```python
from build123d import *

# Parameters (mm, degrees)
SKETCH1_W           = 25
SKETCH1_H           = 25
SKETCH1_W_2         = 22
SKETCH1_H_2         = 22
BOSS_EXTRUDE1_DEPTH = 310
SKETCH2_W           = 25
SKETCH2_H           = 25
SKETCH2_W_2         = 22
SKETCH2_H_2         = 22
BOSS_EXTRUDE2_DEPTH = 30
SKETCH8_R           = 5
CUT_EXTRUDE1_DEPTH  = 25
SKETCH9_R           = 18
SKETCH9_R_2         = 5
BOSS_EXTRUDE3_DEPTH = 10
SKETCH10_R          = 18
SKETCH10_R_2        = 5
BOSS_EXTRUDE4_DEPTH = 10
SKETCH11_W          = 12
SKETCH11_H          = 10
CUT_EXTRUDE2_DEPTH  = 5


with BuildPart() as part:
    # Sketch1 → Boss-Extrude1 (new body)
    with BuildSketch(Plane(origin=(0, 0, 0), x_dir=(1, 0, 0), z_dir=(0, 1, 0))):
        with Locations((30.5, -0.057992327)):
            Rectangle(SKETCH1_W, SKETCH1_H)
        with Locations((30.5, -0.057992327)):
            Rectangle(SKETCH1_W_2, SKETCH1_H_2, mode=Mode.SUBTRACT)
    boss_extrude1 = extrude(amount=BOSS_EXTRUDE1_DEPTH)

    # Sketch2 → Boss-Extrude2 (add)
    # profile 1 of 2: a face of its own
    with BuildSketch(Plane.ZY.offset(-18)):
        with Locations((0.057992327, 197.5)):
            Rectangle(SKETCH2_W, SKETCH2_H)
        with Locations((0.057992327, 197.5)):
            Rectangle(SKETCH2_W_2, SKETCH2_H_2, mode=Mode.SUBTRACT)
    # profile 2 of 2: a face of its own
    with BuildSketch(Plane.ZY.offset(-18)):
        with Locations((0.057992327, 112.5)):
            Rectangle(SKETCH2_W, SKETCH2_H)
        with Locations((0.057992327, 112.5)):
            Rectangle(SKETCH2_W_2, SKETCH2_H_2, mode=Mode.SUBTRACT)
    boss_extrude2 = extrude(amount=BOSS_EXTRUDE2_DEPTH)

    # Sketch8 → Cut-Extrude1 (cut)
    with BuildSketch(Plane.ZY.offset(-18)):
        with Locations((0, 280)):
            Circle(SKETCH8_R)
        with Locations((0, 30)):
            Circle(SKETCH8_R)
    cut_extrude1 = extrude(amount=-CUT_EXTRUDE1_DEPTH, mode=Mode.SUBTRACT)

    # Sketch9 → Boss-Extrude3 (add)
    # profile 1 of 3: a face of its own
    with BuildSketch(Plane(origin=(43, 0, 0), x_dir=(0, 0, -1), z_dir=(1, 0, 0))):
        with Locations((0, 30)):
            Circle(SKETCH9_R)
        with Locations(Location((0, 30, 0), (0, 0, 180))):
            Circle(SKETCH9_R_2, mode=Mode.SUBTRACT)
    # profile 2 of 3: a face of its own
    with BuildSketch(Plane(origin=(43, 0, 0), x_dir=(0, 0, -1), z_dir=(1, 0, 0))):
        with BuildLine():
            Line((-6, 13.029437252), (-6, 3.029437252))
            Line((-6, 3.029437252), (6, 3.029437252))
            Line((6, 3.029437252), (6, 13.029437252))
            ThreePointArc((6, 13.029437252), (0, 12), (-6, 13.029437252))
        make_face()
    # profile 3 of 3: a face of its own
    with BuildSketch(Plane(origin=(43, 0, 0), x_dir=(0, 0, -1), z_dir=(1, 0, 0))):
        with BuildLine():
            Line((-6, 46.970562748), (-6, 56.970562748))
            Line((-6, 56.970562748), (6, 56.970562748))
            Line((6, 56.970562748), (6, 46.970562748))
            ThreePointArc((6, 46.970562748), (0, 48), (-6, 46.970562748))
        make_face()
    boss_extrude3 = extrude(amount=BOSS_EXTRUDE3_DEPTH)

    # Sketch10 → Boss-Extrude4 (add)
    # profile 1 of 3: a face of its own
    with BuildSketch(Plane(origin=(43, 0, 0), x_dir=(0, 0, -1), z_dir=(1, 0, 0))):
        with Locations((0, 280)):
            Circle(SKETCH10_R)
        with Locations(Location((0, 280, 0), (0, 0, 180))):
            Circle(SKETCH10_R_2, mode=Mode.SUBTRACT)
    # profile 2 of 3: a face of its own
    with BuildSketch(Plane(origin=(43, 0, 0), x_dir=(0, 0, -1), z_dir=(1, 0, 0))):
        with BuildLine():
            Line((-6, 296.970562748), (-6, 306.970562748))
            Line((-6, 306.970562748), (6, 306.970562748))
            Line((6, 306.970562748), (6, 296.970562748))
            ThreePointArc((6, 296.970562748), (0, 298), (-6, 296.970562748))
        make_face()
    # profile 3 of 3: a face of its own
    with BuildSketch(Plane(origin=(43, 0, 0), x_dir=(0, 0, -1), z_dir=(1, 0, 0))):
        with BuildLine():
            Line((-6, 263.029437252), (-6, 253.029437252))
            Line((-6, 253.029437252), (6, 253.029437252))
            Line((6, 253.029437252), (6, 263.029437252))
            ThreePointArc((6, 263.029437252), (0, 262), (-6, 263.029437252))
        make_face()
    boss_extrude4 = extrude(amount=BOSS_EXTRUDE4_DEPTH)

    # Sketch11 → Cut-Extrude2 (cut)
    with BuildSketch(Plane(origin=(53, 0, 0), x_dir=(0, 0, -1), z_dir=(1, 0, 0))):
        with Locations((0, 8.029437252)):
            Rectangle(SKETCH11_W, SKETCH11_H)
        with Locations((0, 51.970562748)):
            Rectangle(SKETCH11_W, SKETCH11_H)
        with Locations((0, 258.029437252)):
            Rectangle(SKETCH11_W, SKETCH11_H)
        with Locations((0, 301.970562748)):
            Rectangle(SKETCH11_W, SKETCH11_H)
    cut_extrude2 = extrude(amount=-CUT_EXTRUDE2_DEPTH, mode=Mode.SUBTRACT)

    # Mirror1: Boss-Extrude1, Boss-Extrude2, Cut-Extrude1, Boss-Extrude3, Boss-Extrude4, Cut-Extrude2 across plane
    add(boss_extrude1.mirror(Plane.ZY.offset(12)))
    add(boss_extrude2.mirror(Plane.ZY.offset(12)))
    add(cut_extrude1.mirror(Plane.ZY.offset(12)), mode=Mode.SUBTRACT)
    add(boss_extrude3.mirror(Plane.ZY.offset(12)))
    add(boss_extrude4.mirror(Plane.ZY.offset(12)))
    add(cut_extrude2.mirror(Plane.ZY.offset(12)), mode=Mode.SUBTRACT)


solid = part.part
```
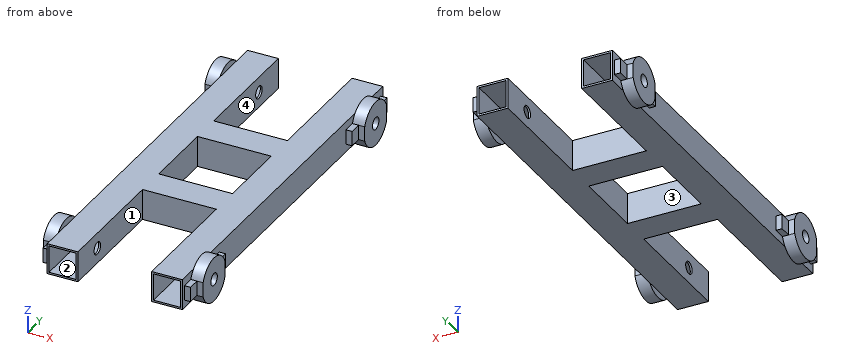
Could you check a few things on this model? Use its own coordinates, in mm. Face numbers are marked on the shaded views. A direction names the side the tool comes from. Coordinates: 2 decimals unless noted, no trailing zeros. Write each loop counter-clockwise with the first axis right and the second up, starting at its lowest first coordinate (ties: lowest second). Pieces come first, ordered by that corner, then holes. Notation, with made-up numbers: (-3.75, -23) -> (47.25, -23) arc R37 ccw to (47.25, 14) -> close; hole circle Ø1 at (58, 20.25). An arc over 180 degrees is marked (long way). Write item = value, one per line. Start each with the question number.
(1) Will these pins go through, and if not, where does the flat tip stop? pin 1 (17.5 mm diameter, centred on y = 196.5, z = 5, fed in from -X); pin 2 (4 mm diameter, centred on x = -33.5, z = 12.5, fed in from -Y); pin 3 (1.5 mm diameter, centred on x = -69.5, z = 0, fed in from +Y).
(2) I want a section at B-B (x = 10.5). Please give me the cut outline in (y, z), plus the area to 3 significant figures.
(3) I need wall thicknesses on line 1 (Y direction, x = -40.5, z = 1); line 2 (X direction, y = 203, z = 5); line 3 (X direction, y = 290, z = 7.5). Which ranges of each line are inside material? Lowest first, please. Write a range as [from, to].
(4) I want a section at A-A (y = 237). Please give me the cut outline in (x, z).
(5) Which directions (+Z, -Z, +X, -X, +Y, -Y) give clear straight access to the entire face, cutting with the end or side of a thin tool? Please do the marked faces 1, 2, 3 and 4.
(6) I want a section at C-C (z = 0). Give the number of separate pieces and of enclosed holes in the cut face, plus the area to 3 significant figures.
Result set:
q1.pin_1 = -67
q1.pin_2 = 100
q1.pin_3 = 306.97
q2.outline = (100, -12.44) -> (125, -12.44) -> (125, 12.56) -> (100, 12.56) -> close; (185, -12.44) -> (210, -12.44) -> (210, 12.56) -> (185, 12.56) -> close; hole (101.5, -10.94) -> (123.5, -10.94) -> (123.5, 11.06) -> (101.5, 11.06) -> close; hole (186.5, -10.94) -> (208.5, -10.94) -> (208.5, 11.06) -> (186.5, 11.06) -> close
q2.area = 282 mm2
q3.line_1 = [100, 101.5], [123.5, 125], [185, 186.5], [208.5, 210]
q3.line_2 = [-67, -65.5], [-43.5, -42], [18, 19.5], [41.5, 43]
q3.line_3 = [-77, -65.5], [-43.5, -42], [18, 19.5], [41.5, 53]
q4.outline = (-67, -12.44) -> (-42, -12.44) -> (-42, 12.56) -> (-67, 12.56) -> close; (18, -12.44) -> (43, -12.44) -> (43, 12.56) -> (18, 12.56) -> close; hole (-65.5, -10.94) -> (-43.5, -10.94) -> (-43.5, 11.06) -> (-65.5, 11.06) -> close; hole (19.5, -10.94) -> (41.5, -10.94) -> (41.5, 11.06) -> (19.5, 11.06) -> close
q5.face_1 = +Z, -Z, -Y
q5.face_2 = +Y, -Y
q5.face_3 = +Z, -Z
q5.face_4 = +Z, -Z, +Y
q6.separate_pieces = 11
q6.enclosed_holes = 3
q6.area = 3,460 mm2
